Could you check a few things on this model? Use its own coordinates, in mm. A direction names the side the tool comes from. Round coordinates to 2 decimals unless told otherwise and drop trailing zeros. Write each loop counter-clockwise with the first axis right and the second up, starting at its lowest first coordinate (ties: lowest second). Pieces come first, ordered by that corner, then holes. Notation, with made-up numbers: (87, -16.5) -> (129, -16.5) arc R28 ccw to (129, 22.5) -> close; hole circle Ø4 at (21.5, 30). An arc over 180 degrees is marked (long way). Answer in a Markdown table with one row per item.
Autodesk Fusion 360 part; units mm, degrees
sketch "Sketch1" plane through (0, 0, 0) normal (1, 0, 0) x (0, 1, 0)
  circle A0 centre (0, 0) radius 35
  dimension "d1" = 70
extrude "Extrude1" add sketch "Sketch1" along normal blind 10 in component "Component"
sketch "Sketch2" plane through (10, 0, 0) normal (1, 0, 0) x (0, 1, 0)
  circle A0 centre (0, 0) radius 35
  circle A1 centre (0, 0) radius 23.5
  dimension "d4" = 47
extrude "Extrude2" add sketch "Sketch2" along normal blind 13 contours A1 in component "Component"
ref_plane "WorkPlane1" through (0, 0, 13) normal (0, 0, 1) x (1, 0, 0)
sketch "Sketch3" plane through (0, 0, 13) normal (0, 0, 1) x (1, 0, 0)
  line L0 (23, 0) -> (23, -35)
  line L1 (23, -35) -> (23, -45)
  line L2 (23, -35) -> (30.3921, -43.8095)
  line L3 (23, -35) -> (34.5, -35) construction
  line L4 (23, 0) -> (60, 0)
  line L5 (23, -23.4992) -> (67, -23.4992)
  line L6 (30.3921, -43.8095) -> (35.3921, -43.8095)
  line L7 (35.3921, -43.8095) -> (52.4344, -23.4992)
  line L8 (35.3921, -43.8095) -> (45, -43.8095)
  line L9 (52.4344, -23.4992) -> (52.4344, 0)
  line L10 (23, 0) -> (23, 35)
  line L11 (23, 35) -> (30.3921, 43.8095)
  line L12 (30.3921, 43.8095) -> (35.3921, 43.8095)
  line L13 (52.4344, 23.4992) -> (52.4344, 0)
  line L14 (35.3921, 43.8095) -> (52.4344, 23.4992)
  dimension "d8" = 35
  dimension "d9" = 10
  dimension "d10" = 50
  dimension "d11" = 11.5
  dimension "d13" = 37
  dimension "d14" = 44
  dimension "d15" = 5
  dimension "d16" = 50
extrude "Extrude3" add sketch "Sketch3" against normal blind 4 in component "Component"
sketch "Sketch4" plane through (0, 0, 13) normal (0, 0, 1) x (-1, 0, 0)
  line L0 (-23, -35) -> (-23, -19.5768)
  line L1 (-23, -19.5768) -> (-23, 19.5768)
  line L2 (-23, 19.5768) -> (-23, 35)
  line L3 (-23, 35) -> (-30.3921, 43.8095)
  line L4 (-30.3921, 43.8095) -> (-35.3921, 43.8095)
  line L5 (-35.3921, 43.8095) -> (-52.4344, 23.4992)
  line L6 (-52.4344, 23.4992) -> (-52.4344, -23.4992)
  line L7 (-52.4344, -23.4992) -> (-35.3921, -43.8095)
  line L8 (-35.3921, -43.8095) -> (-30.3921, -43.8095)
  line L9 (-30.3921, -43.8095) -> (-23, -35)
  line L10 (-32.8921, 43.8095) -> (-32.8921, 40.8095)
  circle A0 centre (-32.8921, 40.8095) radius 1.5
  dimension "d19" = 3
  dimension "d20" = 3
extrude "Extrude4" cut sketch "Sketch4" against normal blind 7 contours A0 in component "Component"
mirror "Mirror1" about plane through (0, 0, 0) normal (0, 1, 0) of "Extrude4" in component "Component"
mirror "Mirror2" about plane through (0, 0, 0) normal (0, 0, 1) of "Extrude3", "Mirror1", "Extrude4" in component "Component"
sketch "Sketch5" plane through (23, 0, 0) normal (1, 0, 0) x (0, 1, 0)
  line L0 (-19.5768, 13) -> (19.5768, 13)
  arc A0 (19.5768, 13) -> (-19.5768, 13) centre (0, 0) ccw
  line L1 (0, 13) -> (0, 23.5)
  line L2 (0, 13) -> (-1, 13)
  line L3 (-1, 13) -> (-1, 22)
  line L4 (-1, 22) -> (1, 22)
  line L5 (1, 22) -> (1, 13)
extrude "Extrude5" add sketch "Sketch5" along normal blind 3 contours L0 L1 L2 L3 L4 | L0 L1 L4 L5 in component "Component"
fillet "Fillet1" radius 1 2 edges at (24.5, 1, 22) (24.5, -1, 22) in component "Component"
mirror "Mirror3" about plane through (0, 0, 0) normal (0, 0, 1) of "Extrude5", "Fillet1" in component "Component"
sketch "Sketch6" plane through (52.4344, 0, 0) normal (1, 0, 0) x (0, 1, 0)
  line L0 (23.4992, 13) -> (-23.4992, 13)
  line L1 (-23.4992, 13) -> (-23.4992, 9)
  line L2 (-23.4992, 9) -> (23.4992, 9)
  line L3 (23.4992, 9) -> (23.4992, 13)
  line L4 (8, -13) -> (-8, -13)
  line L5 (-8, -13) -> (-8, 13)
  line L6 (-8, 13) -> (8, 13)
  line L7 (8, 13) -> (8, -13)
  line L8 (8, -13) -> (-8, 13) construction
  line L9 (-8, -13) -> (8, 13) construction
extrude "Extrude6" add sketch "Sketch6" along normal blind 3 contours L0 L2 L5 L6 L7 | L2 L4 L5 L7 in component "Component"
sketch "Sketch7" plane through (0, 0, 0) normal (-1, 0, 0) x (0, -1, 0)
  circle A0 centre (0, 0) radius 35
  circle A1 centre (0, 0) radius 10
  dimension "d35" = 20
extrude "Extrude7" cut sketch "Sketch7" against normal blind 10 contours A1 in component "Component"
component "Component" placed x (1, 0, 0) y (0, 1, 0) z (0, 0, 1) at (0, 0, 0)
1) For faces 1 (the face through (23, 27, -11)), 2 (the face through (24, -1, -17)), 3 (the face through (54, -8, 0)), which set-ups out of +Z, -Z, +X, -X, +Y, -Y let a thin tool reach every point of the face, with its end or its side?
Findings:
| item | result |
|---|---|
| face 1 | -Z, +Y |
| face 2 | -Z, +X, -Y |
| face 3 | +Z, -Z, +X, -Y |
2) Thinking about a two-plate mould opening in Z: for faces 4 (the face through (23, -27, 11)), 5 (the face through (4.93, 2.17, -9.76)), which applies, +Z half, -Z half, draft (parallel to the pull), parting line (faces both ways), or undercut?
Findings:
| item | result |
|---|---|
| face 4 | draft |
| face 5 | undercut |
3) Imagine slicing it at D-D, the plane z = -18.5. Please give me the cut outline in (x, y).
Findings:
| item | result |
|---|---|
| outline | (0, -29.71) -> (10, -29.71) -> (10, -14.49) -> (23, -14.49) -> (23, -1) -> (26, -1) -> (26, 1) -> (23, 1) -> (23, 14.49) -> (10, 14.49) -> (10, 29.71) -> (0, 29.71) -> close |
4) Please list where these lines run through material, in increasing order: line 1 (Z direction, x = 24, y = -17); line 2 (Y direction, x = 32, z = -9.5); line 3 (Z direction, x = 6, y = 0).
Findings:
| item | result |
|---|---|
| line 1 | z = -13 to -9, 9 to 13 |
| line 2 | y = -43.81 to -42.02, -39.6 to 39.6, 42.02 to 43.81 |
| line 3 | z = -35 to -10, 10 to 35 |
5) Imagine slicing it at A-A, the plane z = 0. Please give me the cut outline in (x, y), plus the area to 3 significant figures.
Findings:
| item | result |
|---|---|
| outline | (0, -35) -> (10, -35) -> (10, -23.5) -> (23, -23.5) -> (23, 23.5) -> (10, 23.5) -> (10, 35) -> (0, 35) -> (0, 10) -> (10, 10) -> (10, -10) -> (0, -10) -> close; (52.43, -8) -> (55.43, -8) -> (55.43, 8) -> (52.43, 8) -> close |
| area | 1,160 mm^2 |
6) Imagine slicing it at C-C, the plane y = 30. Please give me the cut outline in (x, z).
Findings:
| item | result |
|---|---|
| outline | (0, -18.03) -> (10, -18.03) -> (10, 18.03) -> (0, 18.03) -> close; (23, -13) -> (46.98, -13) -> (46.98, -9) -> (23, -9) -> close; (23, 9) -> (46.98, 9) -> (46.98, 13) -> (23, 13) -> close |
7) For pin 1 (3 mm diameter, centred on y = -3.5, z = -17.5, fed in from +X); pin 2 (1 mm diameter, centred on x = 29.5, y = 15.5, fed in from +Z); pin 3 (0.6 mm diameter, centred on y = 0.5, z = 19, fed in from +X); pin 4 (1.5 mm diameter, centred on x = 34, z = 7.5, fed in from +Y), each with a flat end and sliding along its axis, tell me the tip position at first contact or that it passes through.
Findings:
| item | result |
|---|---|
| pin 1 | stops at x = 23 |
| pin 2 | stops at z = 13 |
| pin 3 | stops at x = 26 |
| pin 4 | passes through |
8) Imagine slicing it at B-B, the plane x = 47. Please give me the cut outline in (y, z).
Findings:
| item | result |
|---|---|
| outline | (-29.98, -13) -> (29.98, -13) -> (29.98, -9) -> (-29.98, -9) -> close; (-29.98, 9) -> (29.98, 9) -> (29.98, 13) -> (-29.98, 13) -> close |
